Input: dimensioned drawing with shaded views. Units: mm. Origin: part minimum x, y, z. Round coordinates to 2 decimals unless told otherwise and drop trailing zeros. Loops run counter-clockwise (first coordinate to the right, second up) from the corner with the lowest first, then second, coordinate; pieces in that order, holes last. Notation, with made-up numbers: M 15,-36 L 20,-36 A17 cw 20,-15 Z; hole C 28,-32 d8. An arc over 180 degrees is marked long. One line per item, written item: value.
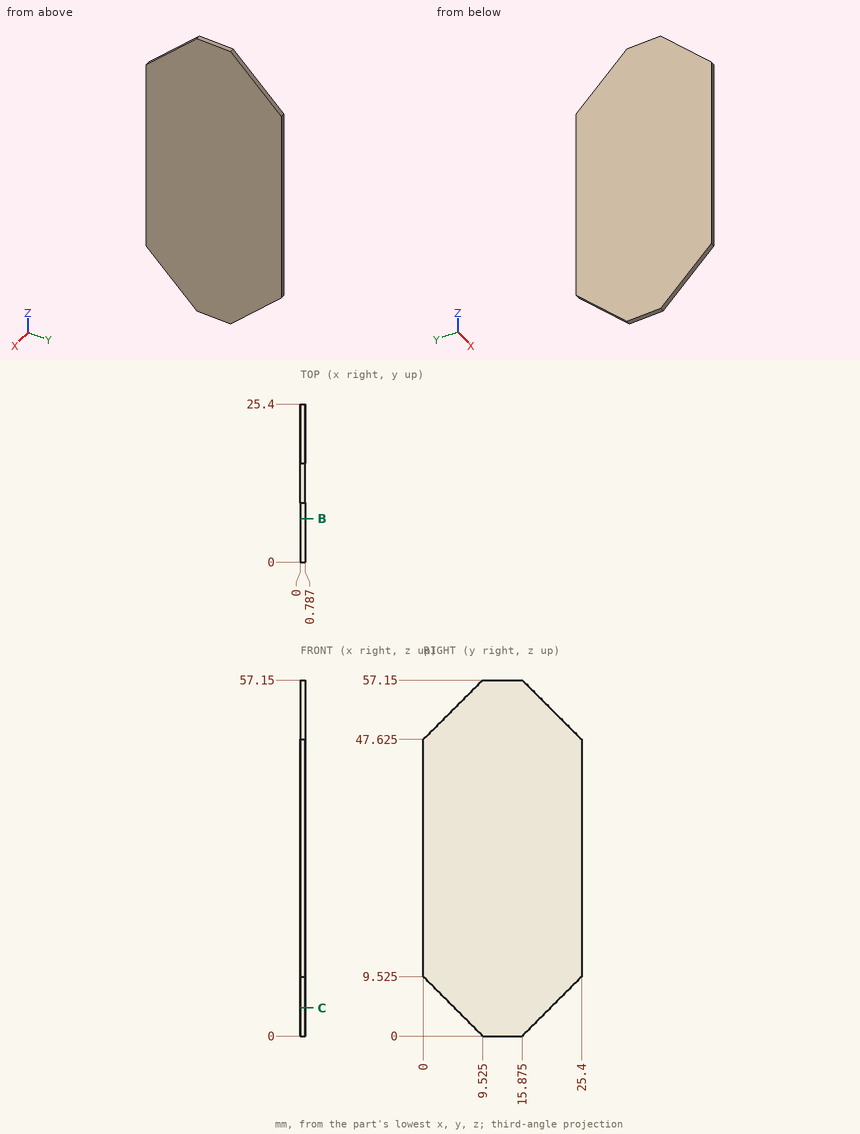
1. Section query B-B (y = 7). Return the cut outline in (x, z) (1 decimal).
Report:
outline: M 0,2.5 L 0.8,2.5 L 0.8,54.6 L 0,54.6 Z
2. Pin query (flat end, axial travel): pin 1 (4 mm diameter, centred on y = 15.5, z = 49.5, fed in from -X). Return the tip coordinate at first contact, or that it passes through.
Report:
pin 1: stops at x = 0
3. Section query C-C (z = 4.5). Return the cut outline in (x, y) (1 decimal).
Report:
outline: M 0,5 L 0.8,5 L 0.8,20.4 L 0,20.4 Z
4. Ray query, line 1 (Z direction, x = 0.55, y = 9) (1 decimal); line 2 (Y direction, x = 0.4, z = 4) (1 decimal); line 3 (Z direction, x = 0.55, y = 22.25) (1 decimal). Return the intervals inside material, ascending. Write a range as [from, to].
Report:
line 1: z = [0.5, 56.6]
line 2: y = [5.5, 19.9]
line 3: z = [6.4, 50.8]
